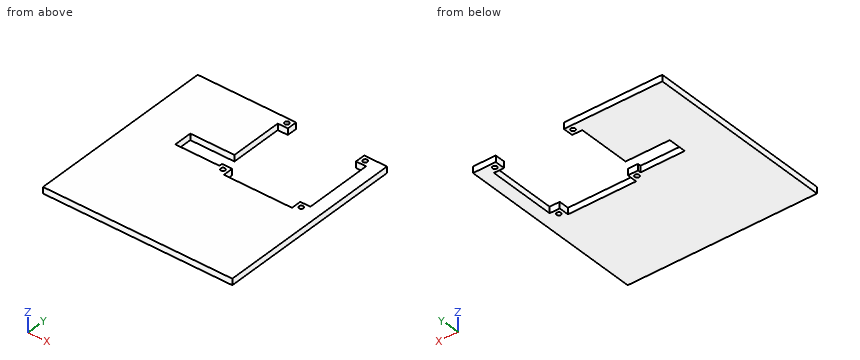
from build123d import *

# Parameters (mm, degrees)
SKETCH1_W           = 150
SKETCH1_H           = 150
BOSS_EXTRUDE1_DEPTH = 5
SKETCH2_R           = 1.75
CUT_EXTRUDE1_DEPTH  = 213.190951739
SKETCH3_W           = 35
SKETCH3_H           = 14.5
CUT_EXTRUDE2_DEPTH  = 213.190951739


with BuildPart() as part:
    # Sketch1 → Boss-Extrude1 (new body)
    with BuildSketch(Plane.XY):
        with Locations((75, 75)):
            Rectangle(SKETCH1_W, SKETCH1_H)
    extrude(amount=BOSS_EXTRUDE1_DEPTH)

    # Sketch2 → Cut-Extrude1 (cut, through all)
    with BuildSketch(Plane.XY.offset(5)):
        with Locations((73.960018565, 84)):
            Circle(SKETCH2_R)
        with Locations((73.960018565, 146)):
            Circle(SKETCH2_R)
        with Locations((135.960018565, 146)):
            Circle(SKETCH2_R)
        with Locations((135.960018565, 84)):
            Circle(SKETCH2_R)
        Polygon((77.960018565, 150), (131.960018565, 150), (131.960018565, 142), (139.960018565, 142), (139.960018565, 88), (131.960018565, 88), (131.960018565, 80), (77.960018565, 80), (77.960018565, 88), (69.960018565, 88), (69.960018565, 142), (77.960018565, 142), align=None)
    extrude(amount=-CUT_EXTRUDE1_DEPTH, mode=Mode.SUBTRACT)

    # Sketch3 → Cut-Extrude2 (cut, through all)
    with BuildSketch(Plane.XY.offset(5)):
        with Locations((52.460018565, 92.75)):
            Rectangle(SKETCH3_W, SKETCH3_H)
    extrude(amount=-CUT_EXTRUDE2_DEPTH, mode=Mode.SUBTRACT)


solid = part.part
The model under review builds one solid part; all positions refer to its coordinate system, in mm. Coordinates: 2 decimals unless noted, no trailing zeros. Write each loop counter-clockwise with the first axis right and the second up, starting at its lowest first coordinate (ties: lowest second). Pieces come first, ordered by that corner, then holes. Notation, with made-up numbers: (2.25, 66.25) -> (7.25, 66.25) arc R19 cw to (7.25, 88.25) -> close; hole circle Ø7 at (-30.75, -16.5). An arc over 180 degrees is marked (long way). Answer in a Markdown table with one row per item.
1. Clearance check with flat-ended pins moving along their axes: pin 1 Ø5.5 at (x, y) = (135.96, 84) entering from -Z; pin 2 Ø2 at (x, y) = (73.96, 84) entering from +Z. State where each tip first meets the part, or that it passes through.
Answers below:
| item | result |
|---|---|
| pin 1 | stops at z = 0 |
| pin 2 | passes through |
2. We need section B-B, the plane y = 146. State the section outline as (x, z) points.
Answers below:
| item | result |
|---|---|
| outline | (0, 0) -> (72.21, 0) -> (72.21, 5) -> (0, 5) -> close; (75.71, 0) -> (77.96, 0) -> (77.96, 5) -> (75.71, 5) -> close; (131.96, 0) -> (134.21, 0) -> (134.21, 5) -> (131.96, 5) -> close; (137.71, 0) -> (150, 0) -> (150, 5) -> (137.71, 5) -> close |
3. Wall thickness on probe 1 along X at (y, z) = (146, 1.6); probe 2 along Y at (x, z) = (60, 2.2); probe 3 along X at (y, z) = (129.5, 0.3): over which ranges is each line inside the solid? List them lowest first. Write a range as [from, to].
Answers below:
| item | result |
|---|---|
| probe 1 | x = [0, 72.21], [75.71, 77.96], [131.96, 134.21], [137.71, 150] |
| probe 2 | y = [0, 85.5], [100, 150] |
| probe 3 | x = [0, 69.96], [139.96, 150] |
4. We need section A-A, the plane y = 131. State the section outline as (x, z) points.
Answers below:
| item | result |
|---|---|
| outline | (0, 0) -> (69.96, 0) -> (69.96, 5) -> (0, 5) -> close; (139.96, 0) -> (150, 0) -> (150, 5) -> (139.96, 5) -> close |
5. We need section C-C, the plane x = 60. State the section outline as (y, z) points.
Answers below:
| item | result |
|---|---|
| outline | (0, 0) -> (85.5, 0) -> (85.5, 5) -> (0, 5) -> close; (100, 0) -> (150, 0) -> (150, 5) -> (100, 5) -> close |
6. We need section D-D, the plane z = 1.05. State the section outline as (x, y) points.
Answers below:
| item | result |
|---|---|
| outline | (0, 0) -> (150, 0) -> (150, 150) -> (131.96, 150) -> (131.96, 142) -> (139.96, 142) -> (139.96, 88) -> (131.96, 88) -> (131.96, 80) -> (77.96, 80) -> (77.96, 88) -> (69.96, 88) -> (69.96, 85.5) -> (34.96, 85.5) -> (34.96, 100) -> (69.96, 100) -> (69.96, 142) -> (77.96, 142) -> (77.96, 150) -> (0, 150) -> close; hole circle Ø3.5 at (73.96, 84); hole circle Ø3.5 at (73.96, 146); hole circle Ø3.5 at (135.96, 84); hole circle Ø3.5 at (135.96, 146) |
